For this review, take the finished solid that the model builds, in its own axes (mm). A direction names the side the tool comes from. Give positions to 0.01 mm unless a question says otherwise; leave off trailing zeros. Loops run counter-clockwise (first coordinate to the right, second up) from the corner with the lowest first, then second, coordinate; pieces in that order, holes last.
```python
from build123d import *

# Parameters (mm, degrees)
SKETCH_1_W          = 82
SKETCH_1_H          = 30
EXTRUDE_1_DEPTH     = 8
SKETCH_2_R          = 2
CUT_EXTRUDE_1_DEPTH = 8
SKETCH_4_W          = 8
SKETCH_4_H          = 30
EXTRUDE_2_DEPTH     = 45
EXTRUDE_5_DEPTH     = 30
SKETCH_15_R         = 2.1
CUT_EXTRUDE_2_DEPTH = 10
SKETCH_17_W         = 37
SKETCH_17_H         = 3
EXTRUDE_6_DEPTH     = 20
EXTRUDE_6_2_DEPTH   = 20
SKETCH_18_W         = 66
SKETCH_18_H         = 36
EXTRUDE_7_DEPTH     = 5
SKETCH_19_W         = 37
SKETCH_19_H         = 3
EXTRUDE_8_DEPTH     = 8
SKETCH_20_W         = 22
SKETCH_20_H         = 3.5
CUT_EXTRUDE_3_DEPTH = 5
SKETCH_21_R         = 16.5
SKETCH_21_R_2       = 13.5
EXTRUDE_9_DEPTH     = 10
SKETCH_22_W         = 9.765091575
SKETCH_22_H         = 3
CUT_EXTRUDE_4_DEPTH = 10
EXTRUDE_10_DEPTH    = 10
SKETCH_24_R         = 1.5
CUT_EXTRUDE_5_DEPTH = 15


with BuildPart() as part:
    # Sketch 1 → Extrude 1 (new body)
    with BuildSketch(Plane(origin=(0, 0, 0), x_dir=(1, 0, 0), z_dir=(0, 1, 0))):
        with Locations((41, 15)):
            Rectangle(SKETCH_1_W, SKETCH_1_H)
    extrude(amount=EXTRUDE_1_DEPTH)

    # Sketch 2 → Cut-Extrude 1 (cut)
    with BuildSketch(Plane(origin=(0, 8, 0), x_dir=(1, 0, 0), z_dir=(0, 1, 0))):
        with Locations(Location((74, 20, 0), (0, 0, 270))):
            Circle(SKETCH_2_R)
        with Locations(Location((74, 10, 0), (0, 0, 270))):
            Circle(SKETCH_2_R)
        with Locations(Location((24.8, 20, 0), (0, 0, 270))):
            Circle(SKETCH_2_R)
        with Locations(Location((24.8, 10, 0), (0, 0, 270))):
            Circle(SKETCH_2_R)
        with BuildLine():
            Line((28.8, 25.5), (70.8, 25.5))
            Line((70.8, 25.5), (70.8, 17.5))
            add(Edge.make_bspline(
                [(70.8, 12.5), (75.8, 12.5), (75.8, 15), (75.8, 17.5), (70.8, 17.5)],
                knots=[4.71238898, 4.71238898, 4.71238898, 6.283185307, 6.283185307, 7.853981634, 7.853981634, 7.853981634], degree=2, weights=[1, 0.707106781, 1, 0.707106781, 1]))
            Line((70.8, 12.5), (70.8, 4.5))
            Line((70.8, 4.5), (28.8, 4.5))
            Line((28.8, 4.5), (28.8, 12.5))
            add(Edge.make_bspline(
                [(28.8, 17.5), (23.8, 17.5), (23.8, 15), (23.8, 12.5), (28.8, 12.5)],
                knots=[1.570796327, 1.570796327, 1.570796327, 3.141592654, 3.141592654, 4.71238898, 4.71238898, 4.71238898], degree=2, weights=[1, 0.707106781, 1, 0.707106781, 1]))
            Line((28.8, 17.5), (28.8, 25.5))
        make_face()
    extrude(amount=-CUT_EXTRUDE_1_DEPTH, mode=Mode.SUBTRACT)

    # Sketch 4 → Extrude 2 (add)
    with BuildSketch(Plane(origin=(0, 8, 0), x_dir=(1, 0, 0), z_dir=(0, 1, 0))):
        with Locations((-4, 15)):
            Rectangle(SKETCH_4_W, SKETCH_4_H)
    extrude(amount=-EXTRUDE_2_DEPTH)

    # Sketch 14 → Extrude 5 (add)
    with BuildSketch(Plane.XY):
        Polygon((0, 0), (0, -2), (2, 0), align=None)
    extrude(amount=-EXTRUDE_5_DEPTH)

    # Sketch 15 → Cut-Extrude 2 (cut)
    with BuildSketch(Plane(origin=(0, 0, 0), x_dir=(0, 0, -1), z_dir=(1, 0, 0))):
        with Locations((7, -33)):
            Circle(SKETCH_15_R)
        with Locations((7, -11)):
            Circle(SKETCH_15_R)
        with Locations((23, -11)):
            Circle(SKETCH_15_R)
        with Locations((23, -33)):
            Circle(SKETCH_15_R)
    extrude(amount=-CUT_EXTRUDE_2_DEPTH, mode=Mode.SUBTRACT)



with BuildPart() as body_2:
    # Sketch 17 → Extrude 6 (new body)
    with BuildSketch(Plane(origin=(0, 8, 0), x_dir=(1, 0, 0), z_dir=(0, 1, 0))):
        with Locations((10.5, -1.5)):
            Rectangle(SKETCH_17_W, SKETCH_17_H)
    extrude(amount=EXTRUDE_6_DEPTH)



with BuildPart() as body_3:
    # Sketch 17 → Extrude 6 2 (new body)
    with BuildSketch(Plane(origin=(0, 8, 0), x_dir=(1, 0, 0), z_dir=(0, 1, 0))):
        with Locations((10.5, 31.5)):
            Rectangle(SKETCH_17_W, SKETCH_17_H)
    extrude(amount=EXTRUDE_6_2_DEPTH)


with BuildPart() as body_2_1:
    add(body_2.part)

    add(body_3.part)  # Extrude 7 merges body 3
    # Sketch 18 → Extrude 7 (add)
    with BuildSketch(Plane(origin=(0, 28, 0), x_dir=(1, 0, 0), z_dir=(0, 1, 0))):
        with Locations((25, 15)):
            Rectangle(SKETCH_18_W, SKETCH_18_H)
    extrude(amount=EXTRUDE_7_DEPTH)


with BuildPart() as part_1:
    add(part.part)

    add(body_2_1.part)  # Extrude 8 merges body 2
    # Sketch 19 → Extrude 8 (add)
    with BuildSketch(Plane(origin=(0, 8, 0), x_dir=(-1, 0, 0), z_dir=(0, -1, 0))):
        with Locations((-10.5, -1.5)):
            Rectangle(SKETCH_19_W, SKETCH_19_H)
        with Locations((-10.5, 31.5)):
            Rectangle(SKETCH_19_W, SKETCH_19_H)
    extrude(amount=EXTRUDE_8_DEPTH)

    # Sketch 20 → Cut-Extrude 3 (cut)
    with BuildSketch(Plane(origin=(0, 33, 0), x_dir=(1, 0, 0), z_dir=(0, 1, 0))):
        with Locations((47, 31.25)):
            Rectangle(SKETCH_20_W, SKETCH_20_H)
        with Locations((47, -1.25)):
            Rectangle(SKETCH_20_W, SKETCH_20_H)
    extrude(amount=-CUT_EXTRUDE_3_DEPTH, mode=Mode.SUBTRACT)



with BuildPart() as body_2_2:
    # Sketch 21 → Extrude 9 (new body)
    with BuildSketch(Plane(origin=(58, 0, 0), x_dir=(0, 0, -1), z_dir=(1, 0, 0))):
        with Locations((14.274721253, 51.113330164)):
            Circle(SKETCH_21_R)
        with Locations((14.274721253, 51.113330164)):
            Circle(SKETCH_21_R_2, mode=Mode.SUBTRACT)
    extrude(amount=-EXTRUDE_9_DEPTH)

    # Sketch 22 → Cut-Extrude 4 (cut)
    with BuildSketch(Plane(origin=(58, 0, 0), x_dir=(0, 0, -1), z_dir=(1, 0, 0))):
        with Locations((-2.130977474, 53.296710416)):
            Rectangle(SKETCH_22_W, SKETCH_22_H)
    extrude(amount=-CUT_EXTRUDE_4_DEPTH, mode=Mode.SUBTRACT)


with BuildPart() as part_2:
    add(part_1.part)

    add(body_2_2.part)  # Extrude 10 merges body 2 2
    # Sketch 23 → Extrude 10 (add)
    with BuildSketch(Plane(origin=(58, 0, 0), x_dir=(0, 0, -1), z_dir=(1, 0, 0))):
        Polygon((-1.808894943, 54.796710416), (-5.808894943, 54.796710416), (-5.808894943, 57.796710416), (0.5, 60.19666955), align=None)
        Polygon((-2.211120899, 51.796710416), (-6.211120899, 51.796710416), (-6.211120899, 48.796710416), (-2.061841205, 48.796710416), align=None)
        Polygon((0.5, 42.029990777), (0.5, 33), (29.5, 33), (29.5, 44.75401518), (27.62078064, 41.411129443), (13.64058676, 34.62552032), align=None)
    extrude(amount=-EXTRUDE_10_DEPTH)

    # Sketch 24 → Cut-Extrude 5 (cut)
    with BuildSketch(Plane(origin=(0, 48.796710416, 0), x_dir=(-1, 0, 0), z_dir=(0, -1, 0))):
        with Locations(Location((-53, -3.931120899, 0), (0, 0, 90))):
            Circle(SKETCH_24_R)
    extrude(amount=-CUT_EXTRUDE_5_DEPTH, mode=Mode.SUBTRACT)


solid = part_2.part
```
Q1. For pin 1 Ø1.5 at (x, z) = (68.5, -4) entering from +Y; pin 2 Ø1.5 at (x, z) = (2, -29) entering from +Y; pin 3 Ø10 at (x, y) = (46, 8) entering from -Z; pin 4 Ø3.5 at (x, z) = (74, -10) entering from +Y, all flat-tipped, find the tip position at first contact; note any pin that passes through.
Answers:
pin 1: stops at y = 8
pin 2: stops at y = 33
pin 3: stops at z = -30
pin 4: passes through
Q2. Consider section B-B on y = -33. Give the boundary of the cut face in (x, z).
Answers:
outline: (-8, -30) - (0, -30) - (0, -25.1) - (-8, -25.1) - close; (-8, -20.9) - (0, -20.9) - (0, -9.1) - (-8, -9.1) - close; (-8, -4.9) - (0, -4.9) - (0, 0) - (-8, 0) - close
Q3. Consider section C-C on y = 25. Give the boundary of the cut face in (x, z), plus the area to 3 significant figures.
Answers:
outline: (-8, -33) - (29, -33) - (29, -30) - (-8, -30) - close; (-8, 0) - (29, 0) - (29, 3) - (-8, 3) - close
area: 222 mm2
Q4. For probe 1 along X at (y, z) = (3.5, -10); probe 2 along Y at (x, z) = (-5, -7); probe 3 along Y at (x, z) = (3, -3), list the stretches that pass through material, from the lowest coordinate up.
Answers:
probe 1: x = -8 to 22.8, 26.8 to 28.8, 70.8 to 72, 76 to 82
probe 2: y = -37 to -35.1, -30.9 to -13.1, -8.9 to 8, 28 to 33
probe 3: y = 0 to 8, 28 to 33
Q5. Mouldability with a two-part tool opening along X and no side actions: class faces 1 (the cylindrical face through (76, 4, -10)), 2 (the flat face through (82, 4, -15)), 3 (the flat face through (53, 54.797, 2)) as +X half, -X half, draft (parallel to the pull), parting line (faces both ways), or undercut.
Answers:
face 1: undercut
face 2: +X half
face 3: draft
Q6. Consider section D-D on z = -6.5. Count the separate pieces of the cut face and the enclosed holes in it, plus the area to 3 significant figures.
Answers:
separate pieces: 6
enclosed holes: 0
area: 1,050 mm2
Q7. Machinability: for faces 4 (the flat face through (55, 4, -30)), 5 (the flat face through (26, 8, -12)), 6 (the flat face through (50, 34, -29.5)), which of the approach directions +Z, -Z, +X, -X, +Y, -Y give a long, thin tool a straight path to every point of the face, cutting with its end or side? Answer none if there is none.
Answers:
face 4: -Z, +X, -Y
face 5: +X, -X
face 6: -Z, +X
Q8. Consider section A-A on x = 46.5. Give the boundary of the cut face in (y, z), plus the area to 3 significant figures.
Answers:
outline: (0, -30) - (8, -30) - (8, -25.5) - (0, -25.5) - close; (0, -4.5) - (8, -4.5) - (8, 0) - (0, 0) - close; (28, -29.5) - (33, -29.5) - (33, -0.5) - (28, -0.5) - close
area: 217 mm2
